from build123d import *

# Parameters (mm, degrees)
SKETCH2_R          = 6
CUT_EXTRUDE1_DEPTH = 8
CUT_EXTRUDE2_DEPTH = 51.955863315
CIRPATTERN1_COUNT  = 6


with BuildPart() as part:
    # Sketch1 → Revolve1 (revolve)
    with BuildSketch(Plane.XY, mode=Mode.PRIVATE) as revolve1_sk:
        with BuildLine():
            Line((0, 0), (11, 0))
            Line((11, 0), (11, -10))
            ThreePointArc((11, -10), (10.196152423, -13), (8, -15.196152423))
            Line((8, -15.196152423), (11, -15.196152423))
            ThreePointArc((11, -15.196152423), (12.5, -16.696152423), (11, -18.196152423))
            Line((11, -18.196152423), (8, -18.196152423))
            ThreePointArc((8, -18.196152423), (8.648844598, -22.489085058), (10.5, -26.416360653))
            ThreePointArc((10.5, -26.416360653), (13.000170941, -34.708180327), (10.5, -43))
            Line((10.5, -43), (14, -43))
            ThreePointArc((14, -43), (15.5, -44.5), (14, -46))
            Line((14, -46), (0, -46))
            Line((0, -46), (0, 0))
        make_face()
    revolve(revolve1_sk.sketch.rotate(Axis((0, 0, 0), (0, -1, 0)), 90), axis=Axis((0, 0, 0), (0, -1, 0)))

    # Sketch2 → Cut-Extrude1 (cut)
    with BuildSketch(Plane(origin=(0, 0, 0), x_dir=(1, 0, 0), z_dir=(0, 1, 0))):
        with Locations(Location((0, 0, 0), (0, 0, 270))):
            Circle(SKETCH2_R)
    extrude(amount=-CUT_EXTRUDE1_DEPTH, mode=Mode.SUBTRACT)

    # Sketch3 → Cut-Extrude2 (cut, symmetric)
    with BuildSketch(Plane.XY):
        Polygon((-2.646002044, 0), (-1.648690033, -4), (1.648690033, -4), (2.353997956, 0), align=None)
    cut_extrude2 = extrude(amount=CUT_EXTRUDE2_DEPTH, both=True, mode=Mode.SUBTRACT)

    # CirPattern1: Cut-Extrude2 ×6 about axis
    cirpattern1_axis = Axis((0, 0, 0), (0, 1, 0))
    for i in range(1, CIRPATTERN1_COUNT):
        add(cut_extrude2.rotate(cirpattern1_axis, i * 360 / CIRPATTERN1_COUNT), mode=Mode.SUBTRACT)


solid = part.part
Input: part model. Units: mm. Frame: model coordinates. A direction names the side the tool comes from. Coordinates: 2 decimals unless noted, no trailing zeros. Loops run counter-clockwise (first coordinate to the right, second up) from the corner with the lowest first, then second, coordinate; pieces in that order, holes last.
Q1. Contact query for flat-ended pins moving along their axis: pin 1 (1 mm diameter, centred on x = 0, z = -9, fed in from +Y); pin 2 (3.5 mm diameter, centred on x = -0.5, z = 1, fed in from +Y); pin 3 (12 mm diameter, centred on x = -7.5, y = -15.5, fed in from -Z) (3 decimals). Output: stop coordinate, or through.
Q2. Set-up query: faces 1 (the face through (-5.93, -1.97, 5.91)), 2 (the face through (-9.4, -43, -5.1)), 3 (the face through (-2.154, -1.972, -8.092)), 4 (the face through (-8.152, -1.972, 2.219)). Return all of +Z, -Z, +X, -X, +Y, -Y with unobstructed straight access to the full face (end or side cutting, diameter ignored); none if empty.
Q3. Cut plane C-C (y = -23). Output: boundary loops of the cut face in (x, z).
Q4. Cut plane A-A (y = -7). Output: boundary loops of the cut face in (x, z).
Q5. Cut plane B-B (z = -8.5). Give the number of separate pieces and of enclosed holes in the cut face, then the cut area to 3 significant figures.
Q6. Draft query along X for faces 5 (the face through (2.154, -1.972, 8.092)), 6 (the face through (0, -46, 0)), 7 (the face through (-6, -1.97, -5.95)). Return one class per face: +X half, -X half, draft (parallel to the pull), parting line (faces both ways), or undercut.
Q7. Material intervals for line 1 (Y direction, x = -5, z = -10); line 2 (X direction, y = -4.25, z = 0); line 3 (Y direction, x = 0.5, z = -5), sorted ascending.
Working result:
1. pin 1: stops at y = -4
1. pin 2: stops at y = -8
1. pin 3: stops at z = -12.395
2. face 1: -X, +Y
2. face 2: none
2. face 3: +Z, -Z, +Y
2. face 4: +Y
3. outline: circle Ø17.63 at (0, 0)
4. outline: circle Ø22 at (0, 0); hole circle Ø12 at (0, 0)
5. separate pieces: 3
5. enclosed holes: 0
5. area: 626 mm2
6. face 5: undercut
6. face 6: draft
6. face 7: -X half
7. line 1: y = -46 to -43, -41.87 to -27.55, -18.19 to -15.21
7. line 2: x = -11 to -6, 6 to 11
7. line 3: y = -46 to -8
